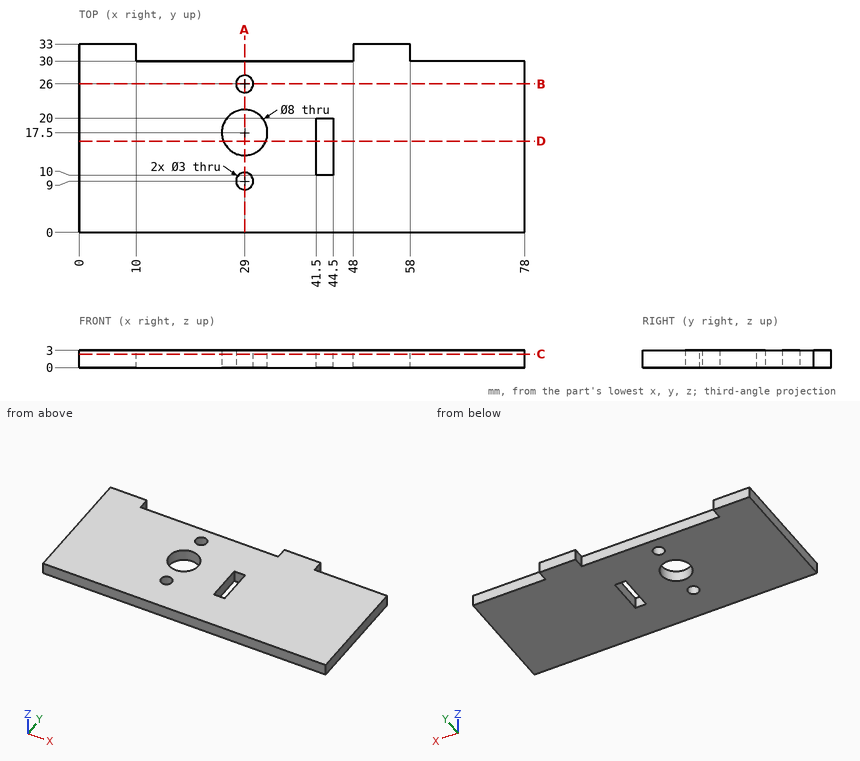
Design review of the part shown in the three views and the two pictorial views. Dimensions are in mm from the part's minimum x, y and z. Round coordinates to 2 decimals unless told otherwise and drop trailing zeros. Loops run counter-clockwise (first coordinate to the right, second up) from the corner with the lowest first, then second, coordinate; pieces in that order, holes last. Notation, with made-up numbers: (-39, 66) -> (-2, 66) arc R38 ccw to (-2, 104) -> close; hole circle Ø10 at (65.5, 5). An arc over 180 degrees is marked (long way). Answer as a JSON object with one key per item and string values. Group by question number.
1) For line 1 (Y direction, x = 29, z = 0.85); line 2 (X direction, y = 13, z = 2.1); line 3 (X direction, y = 31.5, z = 2.85), list the stretches that pass through material, from the lowest coordinate up. Write a range as [from, to].
2) We need section A-A on x = 29. Write out the cut boundary in (y, z).
3) We need section B-B on y = 26. Write out the cut boundary in (x, z).
4) We need section D-D on y = 16. Write out the cut boundary in (x, z), then the cut area to 3 significant figures.
5) We need section C-C on z = 2.35. Write out the cut boundary in (x, y), then the cut area to 3 significant figures.
6) For pin 1 Ø1.5 at (x, z) = (65.5, 2) entering from +Y; pin 2 Ø1.5 at (y, z) = (31.5, 2) entering from +X, all flat-tipped, find the tip position at first contact; note any pin that passes through.
Result set:
{
 "1": {"line 1": "[0, 7.5], [10.5, 13.5], [21.5, 24.5], [27.5, 30]", "line 2": "[0, 41.5], [44.5, 78]", "line 3": "[0, 10], [48, 58]"},
 "2": {"outline": "(0, 0) -> (7.5, 0) -> (7.5, 3) -> (0, 3) -> close; (10.5, 0) -> (13.5, 0) -> (13.5, 3) -> (10.5, 3) -> close; (21.5, 0) -> (24.5, 0) -> (24.5, 3) -> (21.5, 3) -> close; (27.5, 0) -> (30, 0) -> (30, 3) -> (27.5, 3) -> close"},
 "3": {"outline": "(0, 0) -> (27.5, 0) -> (27.5, 3) -> (0, 3) -> close; (30.5, 0) -> (78, 0) -> (78, 3) -> (30.5, 3) -> close"},
 "4": {"outline": "(0, 0) -> (25.29, 0) -> (25.29, 3) -> (0, 3) -> close; (32.71, 0) -> (41.5, 0) -> (41.5, 3) -> (32.71, 3) -> close; (44.5, 0) -> (78, 0) -> (78, 3) -> (44.5, 3) -> close", "area": "203 mm²"},
 "5": {"outline": "(0, 0) -> (78, 0) -> (78, 30) -> (58, 30) -> (58, 33) -> (48, 33) -> (48, 30) -> (10, 30) -> (10, 33) -> (0, 33) -> close; hole circle Ø8 at (29, 17.5); hole circle Ø3 at (29, 9); hole circle Ø3 at (29, 26); hole (41.5, 10) -> (44.5, 10) -> (44.5, 20) -> (41.5, 20) -> close", "area": "2,310 mm²"},
 "6": {"pin 1": "y = 30", "pin 2": "x = 58"}
}
